from build123d import *

# Parameters (mm, degrees)
SKETCH1_R           = 6
BOSS_EXTRUDE1_DEPTH = 10
BOSS_EXTRUDE2_START = 10
SKETCH1_3_R         = 6
BOSS_EXTRUDE2_DEPTH = 6
BOSS_EXTRUDE3_START = 16
BOSS_EXTRUDE3_DEPTH = 85
SKETCH3_R           = 2
CUT_EXTRUDE1_DEPTH  = 3
CUT_EXTRUDE7_START  = -3
SKETCH3_8_R         = 2
SKETCH3_8_R_2       = 3
CUT_EXTRUDE7_DEPTH  = 6
CUT_EXTRUDE8_START  = -3
SKETCH3_11_R        = 3
SKETCH3_11_R_2      = 2
CUT_EXTRUDE8_DEPTH  = 16
CIRPATTERN1_COUNT   = 3
SKETCH4_R           = 2
CUT_EXTRUDE9_DEPTH  = 16
BOSS_EXTRUDE4_DEPTH = 30
SKETCH6_R           = 2
CUT_EXTRUDE10_DEPTH = 30
SKETCH8_R           = 2
CUT_EXTRUDE11_DEPTH = 30
CUT_EXTRUDE12_START = 13
SKETCH1_5_R         = 9.6
SKETCH1_5_R_2       = 8.6
SKETCH1_5_R_3       = 6
CUT_EXTRUDE12_DEPTH = 3
CUT_EXTRUDE13_START = 9
SKETCH1_6_R         = 8.6
SKETCH1_6_R_2       = 6
CUT_EXTRUDE13_DEPTH = 7


with BuildPart() as part:
    # Sketch1 → Boss-Extrude1 (new body)
    with BuildSketch(Plane(origin=(0, 0, 0), x_dir=(1, 0, 0), z_dir=(0, 1, 0))):
        Polygon((-11.267949192, 69.494446501), (-65.817930688, -24.988893001), (-54.549981495, -44.505553499), (54.549981495, -44.505553499), (65.817930688, -24.988893001), (11.267949192, 69.494446501), align=None)
        with Locations(Location((0, 0, 0), (0, 0, 270))):
            Circle(SKETCH1_R, mode=Mode.SUBTRACT)
    extrude(amount=BOSS_EXTRUDE1_DEPTH)

    # Sketch1<3> → Boss-Extrude2 (add)
    with BuildSketch(Plane(origin=(0, 0, 0), x_dir=(1, 0, 0), z_dir=(0, 1, 0)).offset(BOSS_EXTRUDE2_START)):
        Polygon((24, 75.494446501), (-24, 75.494446501), (-24, 53.441887617), (-69.282032303, -24.988893001), (-56.282032303, -47.505553499), (56.282032303, -47.505553499), (69.282032303, -24.988893001), (24, 53.441887617), align=None)
        with Locations(Location((0, 0, 0), (0, 0, 270))):
            Circle(SKETCH1_3_R, mode=Mode.SUBTRACT)
    extrude(amount=BOSS_EXTRUDE2_DEPTH)

    # Sketch1<4> → Boss-Extrude3 (add)
    with BuildSketch(Plane(origin=(0, 0, 0), x_dir=(1, 0, 0), z_dir=(0, 1, 0)).offset(BOSS_EXTRUDE3_START)):
        Polygon((24, 75.494446501), (-24, 75.494446501), (-24, 53.441887617), (-41.141016151, 23.75277675), (-69.282032303, -24.988893001), (-56.282032303, -47.505553499), (0, -47.505553499), (56.282032303, -47.505553499), (69.282032303, -24.988893001), (41.141016151, 23.75277675), (24, 53.441887617), align=None)
        Polygon((-21.4, 51.945219717), (-21.4, 57.945219717), (-21.4, 72.894446501), (21.4, 72.894446501), (21.4, 57.945219717), (21.4, 51.945219717), (38.54293994, 22.25277675), (65.817930688, -24.988893001), (54.549981495, -44.505553499), (0, -44.505553499), (-54.549981495, -44.505553499), (-65.817930688, -24.988893001), (-38.54293994, 22.25277675), align=None, mode=Mode.SUBTRACT)
    extrude(amount=BOSS_EXTRUDE3_DEPTH)

    # Sketch3 → Cut-Extrude1 (cut)
    with BuildSketch(Plane(origin=(38.54293994, 0, -22.25277675), x_dir=(-0.5000000000000011, 0, -0.866025403784438), z_dir=(0.8660254037844382, 0, -0.5000000000000011))):
        with Locations((-34.549981495, 5)):
            Circle(SKETCH3_R)
        with Locations((34.549981495, 5)):
            Circle(SKETCH3_R)
    cut_extrude1 = extrude(amount=-CUT_EXTRUDE1_DEPTH, mode=Mode.SUBTRACT)

    # Sketch3<8> → Cut-Extrude7 (cut)
    # profile 1 of 8: a face of its own
    with BuildSketch(Plane(origin=(38.54293994, 0, -22.25277675), x_dir=(-0.5000000000000011, 0, -0.866025403784438), z_dir=(0.8660254037844382, 0, -0.5000000000000011)).offset(CUT_EXTRUDE7_START)):
        Polygon((-32.413785499, 8.7), (-36.686177491, 8.7), (-38.822373487, 5), (-36.686177491, 1.3), (-32.413785499, 1.3), (-30.277589503, 5), align=None)
        with Locations((-34.549981495, 5)):
            Circle(SKETCH3_8_R, mode=Mode.SUBTRACT)
    # profile 2 of 8: a face of its own
    with BuildSketch(Plane(origin=(38.54293994, 0, -22.25277675), x_dir=(-0.5000000000000011, 0, -0.866025403784438), z_dir=(0.8660254037844382, 0, -0.5000000000000011)).offset(CUT_EXTRUDE7_START)):
        Polygon((-38.822373487, 0), (-30.277589503, 0), (-30.277589503, 5), (-32.413785499, 1.3), (-36.686177491, 1.3), (-38.822373487, 5), align=None)
    # profile 3 of 8: a face of its own
    with BuildSketch(Plane(origin=(38.54293994, 0, -22.25277675), x_dir=(-0.5000000000000011, 0, -0.866025403784438), z_dir=(0.8660254037844382, 0, -0.5000000000000011)).offset(CUT_EXTRUDE7_START)):
        Polygon((38.822373487, 5), (36.686177491, 1.3), (32.413785499, 1.3), (30.277589503, 5), (32.413785499, 8.7), (36.686177491, 8.7), align=None)
        with Locations((34.549981495, 5)):
            Circle(SKETCH3_8_R, mode=Mode.SUBTRACT)
    # profile 4 of 8: a face of its own
    with BuildSketch(Plane(origin=(38.54293994, 0, -22.25277675), x_dir=(-0.5000000000000011, 0, -0.866025403784438), z_dir=(0.8660254037844382, 0, -0.5000000000000011)).offset(CUT_EXTRUDE7_START)):
        Polygon((38.822373487, 0), (38.822373487, 5), (36.686177491, 1.3), (32.413785499, 1.3), (30.277589503, 5), (30.277589503, 0), align=None)
    # profile 5 of 8: a face of its own
    with BuildSketch(Plane(origin=(38.54293994, 0, -22.25277675), x_dir=(-0.5000000000000011, 0, -0.866025403784438), z_dir=(0.8660254037844382, 0, -0.5000000000000011)).offset(CUT_EXTRUDE7_START)):
        with Locations((-34.549981495, 5)):
            Circle(SKETCH3_8_R_2)
        with Locations((-34.549981495, 5)):
            Circle(SKETCH3_8_R, mode=Mode.SUBTRACT)
    # profile 6 of 8: a face of its own
    with BuildSketch(Plane(origin=(38.54293994, 0, -22.25277675), x_dir=(-0.5000000000000011, 0, -0.866025403784438), z_dir=(0.8660254037844382, 0, -0.5000000000000011)).offset(CUT_EXTRUDE7_START)):
        with Locations((-34.549981495, 5)):
            Circle(SKETCH3_8_R)
    # profile 7 of 8: a face of its own
    with BuildSketch(Plane(origin=(38.54293994, 0, -22.25277675), x_dir=(-0.5000000000000011, 0, -0.866025403784438), z_dir=(0.8660254037844382, 0, -0.5000000000000011)).offset(CUT_EXTRUDE7_START)):
        with Locations((34.549981495, 5)):
            Circle(SKETCH3_8_R_2)
        with Locations((34.549981495, 5)):
            Circle(SKETCH3_8_R, mode=Mode.SUBTRACT)
    # profile 8 of 8: a face of its own
    with BuildSketch(Plane(origin=(38.54293994, 0, -22.25277675), x_dir=(-0.5000000000000011, 0, -0.866025403784438), z_dir=(0.8660254037844382, 0, -0.5000000000000011)).offset(CUT_EXTRUDE7_START)):
        with Locations((34.549981495, 5)):
            Circle(SKETCH3_8_R)
    cut_extrude7 = extrude(amount=-CUT_EXTRUDE7_DEPTH, mode=Mode.SUBTRACT)

    # Sketch3<11> → Cut-Extrude8 (cut)
    # profile 1 of 4: a face of its own
    with BuildSketch(Plane(origin=(38.54293994, 0, -22.25277675), x_dir=(-0.5000000000000011, 0, -0.866025403784438), z_dir=(0.8660254037844382, 0, -0.5000000000000011)).offset(CUT_EXTRUDE8_START)):
        with Locations((-34.549981495, 5)):
            Circle(SKETCH3_11_R)
        with Locations((-34.549981495, 5)):
            Circle(SKETCH3_11_R_2, mode=Mode.SUBTRACT)
    # profile 2 of 4: a face of its own
    with BuildSketch(Plane(origin=(38.54293994, 0, -22.25277675), x_dir=(-0.5000000000000011, 0, -0.866025403784438), z_dir=(0.8660254037844382, 0, -0.5000000000000011)).offset(CUT_EXTRUDE8_START)):
        with Locations((34.549981495, 5)):
            Circle(SKETCH3_11_R)
        with Locations((34.549981495, 5)):
            Circle(SKETCH3_11_R_2, mode=Mode.SUBTRACT)
    # profile 3 of 4: a face of its own
    with BuildSketch(Plane(origin=(38.54293994, 0, -22.25277675), x_dir=(-0.5000000000000011, 0, -0.866025403784438), z_dir=(0.8660254037844382, 0, -0.5000000000000011)).offset(CUT_EXTRUDE8_START)):
        with Locations((-34.549981495, 5)):
            Circle(SKETCH3_11_R_2)
    # profile 4 of 4: a face of its own
    with BuildSketch(Plane(origin=(38.54293994, 0, -22.25277675), x_dir=(-0.5000000000000011, 0, -0.866025403784438), z_dir=(0.8660254037844382, 0, -0.5000000000000011)).offset(CUT_EXTRUDE8_START)):
        with Locations((34.549981495, 5)):
            Circle(SKETCH3_11_R_2)
    cut_extrude8 = extrude(amount=-CUT_EXTRUDE8_DEPTH, mode=Mode.SUBTRACT)

    # CirPattern1: Cut-Extrude1, Cut-Extrude7, Cut-Extrude8 ×3 about axis
    cirpattern1_axis = Axis((0, 0, 0), (0, 1, 0))
    add([cut_extrude1.rotate(cirpattern1_axis, i * 360 / CIRPATTERN1_COUNT) for i in range(1, CIRPATTERN1_COUNT)], mode=Mode.SUBTRACT)
    add([cut_extrude7.rotate(cirpattern1_axis, i * 360 / CIRPATTERN1_COUNT) for i in range(1, CIRPATTERN1_COUNT)], mode=Mode.SUBTRACT)
    add([cut_extrude8.rotate(cirpattern1_axis, i * 360 / CIRPATTERN1_COUNT) for i in range(1, CIRPATTERN1_COUNT)], mode=Mode.SUBTRACT)

    # Sketch4 → Cut-Extrude9 (cut)
    with BuildSketch(Plane.XY.offset(-72.894446501)):
        with Locations((0, 30)):
            Circle(SKETCH4_R)
        with Locations((0, 96)):
            Circle(SKETCH4_R)
    extrude(amount=-CUT_EXTRUDE9_DEPTH, mode=Mode.SUBTRACT)

    # Sketch5 → Boss-Extrude4 (add)
    with BuildSketch(Plane(origin=(0, 16, 0), x_dir=(1, 0, 0), z_dir=(0, 1, 0))):
        with BuildLine():
            Line((21.4, 51.945219717), (21.4, 21.024747323))
            ThreePointArc((21.4, 21.024747323), (0, -30), (-21.4, 21.024747323))
            Line((-21.4, 21.024747323), (-21.4, 51.945219717))
            Line((-21.4, 51.945219717), (-22.4, 50.213168909))
            Line((-22.4, 50.213168909), (-22.4, 21.429885674))
            ThreePointArc((-22.4, 21.429885674), (0, -31), (22.4, 21.429885674))
            Line((22.4, 21.429885674), (22.4, 50.213168909))
            Line((22.4, 50.213168909), (21.4, 51.945219717))
        make_face()
    extrude(amount=BOSS_EXTRUDE4_DEPTH)

    # Sketch6 → Cut-Extrude10 (cut)
    with BuildSketch(Plane(origin=(41.141016151, 0, -23.75277675), x_dir=(-0.5000000000000007, 0, -0.8660254037844382), z_dir=(0.8660254037844383, 0, -0.5000000000000008))):
        with Locations((-11, 96)):
            Circle(SKETCH6_R)
    cut_extrude10 = extrude(amount=-CUT_EXTRUDE10_DEPTH, mode=Mode.SUBTRACT)

    # Sketch8 → Cut-Extrude11 (cut)
    with BuildSketch(Plane(origin=(0, 0, 44.505553499), x_dir=(-1, 0, 0), z_dir=(0, 0, -1))):
        with Locations((-34.549981495, 96)):
            Circle(SKETCH8_R)
    cut_extrude11 = extrude(amount=-CUT_EXTRUDE11_DEPTH, mode=Mode.SUBTRACT)

    # Mirror1: Cut-Extrude10, Cut-Extrude11 across plane
    add(cut_extrude10.mirror(Plane(origin=(0, 0, 0), x_dir=(0, 0, 1), z_dir=(1, 0, 0))), mode=Mode.SUBTRACT)
    add(cut_extrude11.mirror(Plane(origin=(0, 0, 0), x_dir=(0, 0, 1), z_dir=(1, 0, 0))), mode=Mode.SUBTRACT)

    # Sketch1<5> → Cut-Extrude12 (cut)
    # profile 1 of 2: a face of its own
    with BuildSketch(Plane(origin=(0, 0, 0), x_dir=(1, 0, 0), z_dir=(0, 1, 0)).offset(CUT_EXTRUDE12_START)):
        with Locations(Location((0, 0, 0), (0, 0, 270))):
            Circle(SKETCH1_5_R)
        Circle(SKETCH1_5_R_2, mode=Mode.SUBTRACT)
    # profile 2 of 2: a face of its own
    with BuildSketch(Plane(origin=(0, 0, 0), x_dir=(1, 0, 0), z_dir=(0, 1, 0)).offset(CUT_EXTRUDE12_START)):
        Circle(SKETCH1_5_R_2)
        with Locations(Location((0, 0, 0), (0, 0, 270))):
            Circle(SKETCH1_5_R_3, mode=Mode.SUBTRACT)
    extrude(amount=CUT_EXTRUDE12_DEPTH, mode=Mode.SUBTRACT)

    # Sketch1<6> → Cut-Extrude13 (cut)
    with BuildSketch(Plane(origin=(0, 0, 0), x_dir=(1, 0, 0), z_dir=(0, 1, 0)).offset(CUT_EXTRUDE13_START)):
        with Locations(Location((0, 0, 0), (0, 0, 270))):
            Circle(SKETCH1_6_R)
        with Locations(Location((0, 0, 0), (0, 0, 270))):
            Circle(SKETCH1_6_R_2, mode=Mode.SUBTRACT)
    extrude(amount=CUT_EXTRUDE13_DEPTH, mode=Mode.SUBTRACT)


solid = part.part
Geometry: final body of the model. Coordinates: model frame, mm. A direction names the side the tool comes from. Coordinates: 2 decimals unless noted, no trailing zeros. Order: outer loops, then holes, each group sorted by start corner. A loop starts at its lowest first (then second) coordinate and runs counter-clockwise, first axis right, second up.
(1) Material intervals for probe 1 along Z at (x, y) = (0, 10.05); probe 2 along X at (y, z) = (39.5, 0); probe 3 along X at (y, z) = (61.5, -14), sorted ascending.
(2) Section query C-C (x = 0). State how many separate pieces and enclosed holes the cut face has, plus the area to 3 significant figures.
(3) First-contact query: pin 1 (3 mm diameter, centred on x = -28, y = 66, fed in from -Z); pin 2 (5.5 mm diameter, centred on y = 2, z = 39, fed in from +X); pin 3 (6 mm diameter, centred on y = 63.5, z = 18, fed in from +X). Flat tips, straight axial feed; report the tip coordinate or a pass-through.
(4) Section query A-A (y = 30). Return the cut outline in (x, z).
(5) Section query D-D (z = -61). Return the cut outline in (x, y), plus the area to 3 significant figures.
(6) Draft query along Y for faces 1 (the face through (8.095, 14.479, 5.161)), 2 (the face through (-35, 5, 25.506)), 3 (the face through (49.049, 6.824, 7.859)). Return one class per face: pulls with the +Y half, pulls with the -Y half, needs draft (parallel to the pull), parting line crosses it, or undercut.
(7) Access query for faces 4 (the face through (4.834, 5.042, -42.638)), 5 (the face through (-60.263, 4.93, 34.611)), 6 (the face through (22.4, 31, -36)), 7 (the face through (48.52, 2.47, 6.95)). Directions: +Z, -Z, +X, -X, +Y, -Y. A direction counts if a zero-diameter tool reaches every point of the face in a straight line with its end or side. Return the directions, or none.
Solution:
1. probe 1: z = -75.49 to -8.6, 8.6 to 47.51
1. probe 2: x = -54.85 to -51.39, -31 to -30, 30 to 31, 51.39 to 54.85
1. probe 3: x = -46.77 to -43.31, 43.31 to 46.77
2. separate pieces: 4
2. enclosed holes: 0
2. area: 2,130 mm2
3. pin 1: stops at z = -49.11
3. pin 2: stops at x = 59.32
3. pin 3: stops at x = 66.98
4. outline: (-69.28, 24.99) - (-24, -53.44) - (-24, -75.49) - (-2, -75.49) - (-2, -72.89) - (-21.4, -72.89) - (-21.4, -21.02) arc R30 cw (long way) to (21.4, -21.02) - (21.4, -72.89) - (2, -72.89) - (2, -75.49) - (24, -75.49) - (24, -53.44) - (69.28, 24.99) - (56.28, 47.51) - (-56.28, 47.51) - close; hole (-65.82, 24.99) - (-22.4, -50.21) - (-22.4, -21.43) arc R31 cw (long way) to (22.4, -21.43) - (22.4, -50.21) - (65.82, 24.99) - (54.55, 44.51) - (-54.55, 44.51) - close
5. outline: (-24, 10) - (-16.17, 10) - (-16.17, 0) - (16.17, 0) - (16.17, 10) - (24, 10) - (24, 101) - (21.4, 101) - (21.4, 16) - (-21.4, 16) - (-21.4, 101) - (-24, 101) - close
5. area: 1,050 mm2
6. face 1: needs draft
6. face 2: undercut
6. face 3: pulls with the -Y half
7. face 4: none
7. face 5: +Z, -X, -Y
7. face 6: +Y
7. face 7: -Y
